Autodesk Inventor part; units mm, degrees
ref_plane "YZ Plane" through (0, 0, 0) normal (1, 0, 0) x (0, 1, 0)
ref_plane "XZ Plane" through (0, 0, 0) normal (0, 1, 0) x (-1, 0, 0)
ref_plane "XY Plane" through (0, 0, 0) normal (0, 0, 1) x (1, 0, 0)
sketch "Sketch1" plane through (0, 0, 0) normal (1, 0, 0) x (0, 1, 0)
  line L0 (8, 10) -> (0, 10)
  line L1 (0, 10) -> (0, 40)
  line L2 (0, 40) -> (17.6795, 40)
  arc A0 (65, 50) -> (50, 58.6603) centre (55, 50) ccw
  line L3 (65, 50) -> (65, 40)
  line L4 (61.5, 0) -> (66, 0)
  line L5 (65, 40) -> (65, 30)
  line L6 (65, 30) -> (85, 30)
  line L7 (85, 30) -> (85, 10)
  line L8 (10, 8) -> (10, 0)
  line L9 (50, 58.6603) -> (17.6795, 40)
  circle A1 centre (55, 50) radius 6
  line L10 (85, 10) -> (67, 10)
  line L11 (65, 8) -> (65, 0)
  line L12 (49.5, 10) -> (19.5, 10)
  line L13 (17, 7.5) -> (17, 0)
  line L14 (17, 0) -> (52, 0)
  line L15 (52, 0) -> (52, 7.5)
  arc A2 (67, 10) -> (65, 8) centre (65, 10) ccw
  arc A3 (49.5, 10) -> (52, 7.5) centre (52, 10) ccw
  arc A4 (17, 7.5) -> (19.5, 10) centre (17, 10) ccw
  arc A5 (10, 8) -> (8, 10) centre (10, 10) ccw
  line L16 (65, -40) -> (65, -30)
  arc A6 (52, -7.5) -> (49.5, -10) centre (52, -10) ccw
  line L17 (52, 0) -> (52, -7.5)
  line L18 (65, -50) -> (65, -40)
  arc A7 (50, -58.6603) -> (65, -50) centre (55, -50) ccw
  line L19 (49.5, -10) -> (19.5, -10)
  line L20 (50, -58.6603) -> (17.6795, -40)
  arc A8 (19.5, -10) -> (17, -7.5) centre (17, -10) ccw
  circle A9 centre (55, -50) radius 6
  line L21 (8, -10) -> (0, -10)
  line L22 (0, -10) -> (0, -40)
  line L23 (0, -40) -> (17.6795, -40)
  line L24 (17, -7.5) -> (17, 0)
  arc A10 (8, -10) -> (10, -8) centre (10, -10) ccw
  line L25 (10, -8) -> (10, 0)
  line L26 (65, -30) -> (85, -30)
  line L27 (85, -30) -> (85, -10)
  line L28 (65, -8) -> (65, 0)
  arc A11 (65, -8) -> (67, -10) centre (65, -10) ccw
  line L29 (85, -10) -> (67, -10)
  line L30 (17.6795, 40) -> (28.4601, 40)
  point P0 (0, 0)
  point P1 (0, 0)
  dimension "d21" = 35
  dimension "d22" = 55
  dimension "d23" = 85
  dimension "d24" = 12
  dimension "d25" = 2.5
  dimension "d26" = 20
  dimension "d27" = 80
  dimension "d28" = 20
  dimension "d29" = 100
  dimension "d32" = 30
sketch "Sketch2" plane through (0, 0, 0) normal (1, 0, 0) x (0, 1, 0)
  point P0 (0, 0)
extrude "Extrusion1" add sketch "Sketch1" along normal mid plane 10
properties part number "hw8"
Geometry check sheet. Reference: the model listing, model coordinates, mm. A direction names the side the tool comes from. Coordinates: 2 decimals unless noted, no trailing zeros. Order: outer loops, then holes, each group sorted by start corner. A loop starts at its lowest first (then second) coordinate and runs counter-clockwise, first axis right, second up. Notation, with made-up numbers: (4, 11.5) - (9, 11.5) arc R33 cw to (9, 40.5) - close; hole circle Ø11 at (43.5, 79.5). An arc over 180 degrees is marked (long way). Answer in a Markdown table with one row per item. Add a question column.
1) Cross-section at B-B, the plane y = 55. Record the cut outline in (x, z), then the cut area to 3 significant figures.
2) Cross-section at C-C, the plane y = 69.5. Record the cut outline in (x, z), then the cut area to 3 significant figures.
3) Cross-section at D-D, the plane z = -34. Record the cut outline in (x, y), then the cut area to 3 significant figures.
4) Gauge pin test, flat ends, axial feed: P1, Ø3, axis at x = 3.5, y = 68, coming from the +Z side; P2, Ø3, axis at x = 2, z = 2, coming from the +Y side; P3, Ø5, axis at x = -3.5, y = 70.5, coming from the -Z side; P4, Ø3.5, axis at y = 65, z = -10, coming from the -X side. Record the tip position at first contact, or that the pin passes through.
5) Release check for a two-part mould opening along Y. For faces 4 (the flat face through (0, 52, 0)), 5 (the cylindrical face through (-0.1, 60.1, -58.6)), 6 (the flat face through (0, 85, -20)) record: +Y half, -Y half, draft (parallel to the pull), parting line (faces both ways), or undercut.
6) Cross-section at A-A, the plane x = 3.25. State how many separate pieces and enclosed holes the cut face has, then the cut area to 3 significant figures.
7) Material ranges on line 1 along Z through (x, y) = (-2.25, 55); line 2 along Y through (x, z) = (-2, 34.5); line 3 along Z through (x, y) = (1.25, 18.5), recorded low to high. Write a range as [from, to].
8) Set-up check for faces 1 (the flat face through (0, 35, 10)), 2 (the flat face through (0, 9, -40)), 3 (the flat face through (0, 65, 0)): record each of +Z, -Z, +X, -X, +Y, -Y from which the full face is reachable in a straight line by a thin tool's end or side.
Check result:
| question | item | result |
|---|---|---|
| 1 | outline | (-5, -60) - (5, -60) - (5, -56) - (-5, -56) - close; (-5, -44) - (5, -44) - (5, 44) - (-5, 44) - close; (-5, 56) - (5, 56) - (5, 60) - (-5, 60) - close |
| 1 | area | 960 mm² |
| 2 | outline | (-5, -30) - (5, -30) - (5, -10) - (-5, -10) - close; (-5, 10) - (5, 10) - (5, 30) - (-5, 30) - close |
| 2 | area | 400 mm² |
| 3 | outline | (-5, 0) - (5, 0) - (5, 65) - (-5, 65) - close |
| 3 | area | 650 mm² |
| 4 | P1 | stops at z = 30 |
| 4 | P2 | stops at y = 65 |
| 4 | P3 | stops at z = -30 |
| 4 | P4 | passes through |
| 5 | face 4 | undercut |
| 5 | face 5 | parting line |
| 5 | face 6 | +Y half |
| 6 | separate pieces | 1 |
| 6 | enclosed holes | 3 |
| 6 | area | 6,010 mm² |
| 7 | line 1 | z = [-60, -56], [-44, 44], [56, 60] |
| 7 | line 2 | y = [0, 65] |
| 7 | line 3 | z = [-40.47, -8], [8, 40.47] |
| 8 | face 1 | +X, -X |
| 8 | face 2 | -Z, +X, -X, -Y |
| 8 | face 3 | +X, -X, +Y |
